The model under review builds one solid part; all positions refer to its coordinate system, in mm. Face numbers are marked on the shaded views. Round coordinates to 2 decimals unless told otherwise and drop trailing zeros. Write each loop counter-clockwise with the first axis right and the second up, starting at its lowest first coordinate (ties: lowest second). Pieces come first, ordered by that corner, then holes. Notation, with made-up numbers: (51, 51) -> (93, 51) arc R32 cw to (93, 80) -> close; hole circle Ø9 at (-2, -21.75). An arc over 180 degrees is marked (long way). Answer as a JSON object with one key per item and string values. Group by question number.
1) We need section D-D, the plane x = 23. Write out the cut boundary in (y, z).
2) Insertion check: pin 1 Ø10 at (x, z) = (2, 15) entering from -Y; pin 2 Ø6 at (x, y) = (14.5, -31) entering from +Z; pin 3 Ø11.5 at (x, y) = (35.31, 29.05) entering from +Z. Each pin has a flat end and moves straight along its axis. Give the tip position at first contact, or say it passes through.
3) Mouldability with a two-part tool opening along Y and no side actions: class the marked faces 1, 2 and 3 as pulls with the +Y half, pulls with the -Y half, needs draft (parallel to the pull), parting line crosses it, or undercut.
4) We need section B-B, the plane x = 0. Write out the cut boundary in (y, z), then the cut area to 3 significant figures.
5) We need section C-C, the plane z = 12.75. Write out the cut boundary in (x, y).
6) To check wall thickness, follow probe 1 along Z at (x, y) = (-27.5, 5); probe 2 along Y at (x, z) = (-4.5, 19.5); probe 3 along Y at (x, z) = (0, 18.25). State the ranges of each line that lie inside material, in increasing order. Write a range as [from, to].
7) We need section A-A, the plane y = 0. Write out the cut boundary in (x, z).
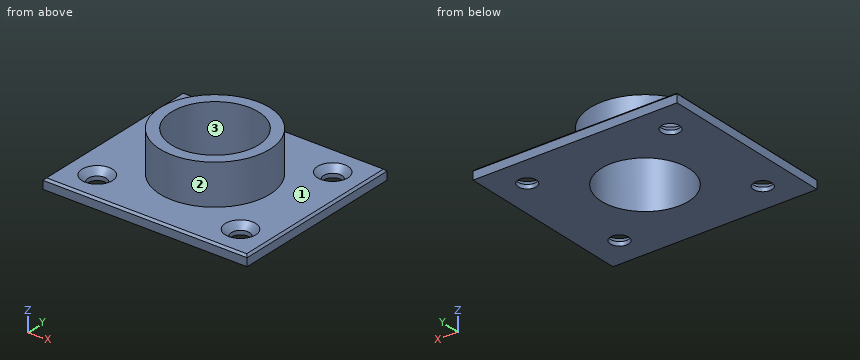
from build123d import *

# Parameters (mm, degrees)
F0_R     = 27.06303
F1_DEPTH = 25
F0_W     = 100.61507
F0_H     = 88.102676
F2_DEPTH = 5
F3_SIZE  = 1
F4_R     = 21.5
F5_DEPTH = 30
F6_R     = 4.5
F7_DEPTH = 12.5
F8_SIZE  = 3


with BuildPart() as f1:
    # F0 (on Top) → F1 (new body)
    with BuildSketch(Plane.XY):
        Circle(F0_R)
    extrude(amount=F1_DEPTH)

    # F0 (on Top) → F2 (join)
    with BuildSketch(Plane.XY):
        Rectangle(F0_W, F0_H)
        Circle(F0_R, mode=Mode.SUBTRACT)
    extrude(amount=F2_DEPTH)

    # F3
    f3_edges = [f1.edges().sort_by_distance(p)[0] for p in [
        (-50.307535, 0, 5),
        (0, -44.051338, 5),
        (50.307535, 0, 5),
        (0, 44.051338, 5),
    ]]
    chamfer(f3_edges, length=F3_SIZE)

    # F4 (on Top) → F5 (cut)
    with BuildSketch(Plane.XY):
        Circle(F4_R)
    extrude(amount=F5_DEPTH, mode=Mode.SUBTRACT)

    # F6 (on Top) → F7 (cut, symmetric)
    with BuildSketch(Plane.XY):
        with Locations((35.307535, -29.051338)):
            Circle(F6_R)
        with Locations((35.307535, 29.051338)):
            Circle(F6_R)
        with Locations((-35.307535, 29.051338)):
            Circle(F6_R)
        with Locations((-35.307535, -29.051338)):
            Circle(F6_R)
    extrude(amount=F7_DEPTH, both=True, mode=Mode.SUBTRACT)

    # F8
    f8_edges = [f1.edges().sort_by_distance(p)[0] for p in [
        (-39.807535, -29.051338, 5),
        (-39.807535, 29.051338, 5),
        (30.807535, 29.051338, 5),
        (30.807535, -29.051338, 5),
    ]]
    chamfer(f8_edges, length=F8_SIZE)


solid = f1.part
Here are the results:
{
 "1": {"outline": "(-44.05, 0) -> (44.05, 0) -> (44.05, 4) -> (43.05, 5) -> (14.26, 5) -> (14.26, 25) -> (-14.26, 25) -> (-14.26, 5) -> (-43.05, 5) -> (-44.05, 4) -> close"},
 "2": {"pin 1": "stops at y = -27.06", "pin 2": "stops at z = 5", "pin 3": "stops at z = 3.25"},
 "3": {"face 1": "needs draft", "face 2": "parting line crosses it", "face 3": "undercut"},
 "4": {"outline": "(-44.05, 0) -> (-21.5, 0) -> (-21.5, 25) -> (-27.06, 25) -> (-27.06, 5) -> (-43.05, 5) -> (-44.05, 4) -> close; (21.5, 0) -> (44.05, 0) -> (44.05, 4) -> (43.05, 5) -> (27.06, 5) -> (27.06, 25) -> (21.5, 25) -> close", "area": "447 mm^2"},
 "5": {"outline": "circle Ø54.13 at (0, 0); hole circle Ø43 at (0, 0)"},
 "6": {"probe 1": "z = [0, 5]", "probe 2": "y = [-26.69, -21.02], [21.02, 26.69]", "probe 3": "y = [-27.06, -21.5], [21.5, 27.06]"},
 "7": {"outline": "(-50.31, 0) -> (-21.5, 0) -> (-21.5, 25) -> (-27.06, 25) -> (-27.06, 5) -> (-49.31, 5) -> (-50.31, 4) -> close; (21.5, 0) -> (50.31, 0) -> (50.31, 4) -> (49.31, 5) -> (27.06, 5) -> (27.06, 25) -> (21.5, 25) -> close"}
}
